Here's how the part is built. I have some questions about the finished solid (model axes, mm). Coordinates: 2 decimals unless noted, no trailing zeros. Loops run counter-clockwise (first coordinate to the right, second up) from the corner with the lowest first, then second, coordinate; pieces in that order, holes last.
from build123d import *

# Parameters (mm, degrees)
SKETCH1_W               = 70
SKETCH1_H               = 100
BOSS_EXTRUDE1_DEPTH     = 1
CUT_EXTRUDE1_DEPTH      = 62.040969848
CUT_EXTRUDE1_DEPTH_BACK = 62.040969848
SKETCH2_R               = 1.7


with BuildPart() as part:
    # Sketch1 → Boss-Extrude1 (new body)
    with BuildSketch(Plane.XY):
        Rectangle(SKETCH1_W, SKETCH1_H)
    extrude(amount=-BOSS_EXTRUDE1_DEPTH)

    # Sketch2 → Cut-Extrude1 (cut, two sides: drawn at the far end of the back side and taken through both)
    with BuildSketch(Plane.XY.offset(-CUT_EXTRUDE1_DEPTH_BACK)):
        with Locations((-30, -35)):
            Circle(SKETCH2_R)
        with Locations((-30, 35)):
            Circle(SKETCH2_R)
        with Locations((30, -35)):
            Circle(SKETCH2_R)
        with Locations((30, 35)):
            Circle(SKETCH2_R)
        with Locations((-15, -40)):
            Circle(SKETCH2_R)
        with Locations((-15, -10)):
            Circle(SKETCH2_R)
        with Locations((-15, 10)):
            Circle(SKETCH2_R)
        with Locations((-15, 40)):
            Circle(SKETCH2_R)
        with Locations((15, -40)):
            Circle(SKETCH2_R)
        with Locations((15, -10)):
            Circle(SKETCH2_R)
        with Locations((15, 10)):
            Circle(SKETCH2_R)
        with Locations((15, 40)):
            Circle(SKETCH2_R)
    extrude(amount=CUT_EXTRUDE1_DEPTH + CUT_EXTRUDE1_DEPTH_BACK, mode=Mode.SUBTRACT)


solid = part.part
Q1. Suppose I cut it at A-A on x = 30. Write out the boundary of the cut face in (y, z), and give its area (3 significant figures).
Q2. Suppose I cut it at B-B on z = -0.7. State how many separate pieces and enclosed holes the cut face has, and give its area (3 significant figures).
Q3. Will this pin go through, and if not, where does the flat tip stop? P1, Ø2.5, axis at x = -15, y = -40, coming from the -Z side.
Q4. Suppose I cut it at C-C on y = 35. Write out the boundary of the cut face in (x, z).
Q5. We'd pull the mould along Y, two halves only. Please class faces 1 (the flat face through (0, 1, -1)), 2 (the cylindrical face through (30.8, 33.5, -0.5)): pulls with the +Y half, pulls with the -Y half, needs draft (parallel to the pull), parting line crosses it, or undercut.
Q6. Suppose I cut it at D-D on x = 15. Write out the boundary of the cut face in (y, z), and give its area (3 significant figures).
Q7. Please list where these lines run through material, in increasing order: probe 1 along Y at (x, z) = (30, -0.4); probe 2 along X at (y, z) = (35, -0.55); probe 3 along Y at (x, z) = (-15, -0.25).
Check values:
1. outline: (-50, -1) - (-36.7, -1) - (-36.7, 0) - (-50, 0) - close; (-33.3, -1) - (33.3, -1) - (33.3, 0) - (-33.3, 0) - close; (36.7, -1) - (50, -1) - (50, 0) - (36.7, 0) - close
1. area: 93.2 mm2
2. separate pieces: 1
2. enclosed holes: 12
2. area: 6,890 mm2
3. P1: passes through
4. outline: (-35, -1) - (-31.7, -1) - (-31.7, 0) - (-35, 0) - close; (-28.3, -1) - (28.3, -1) - (28.3, 0) - (-28.3, 0) - close; (31.7, -1) - (35, -1) - (35, 0) - (31.7, 0) - close
5. face 1: needs draft
5. face 2: undercut
6. outline: (-50, -1) - (-41.7, -1) - (-41.7, 0) - (-50, 0) - close; (-38.3, -1) - (-11.7, -1) - (-11.7, 0) - (-38.3, 0) - close; (-8.3, -1) - (8.3, -1) - (8.3, 0) - (-8.3, 0) - close; (11.7, -1) - (38.3, -1) - (38.3, 0) - (11.7, 0) - close; (41.7, -1) - (50, -1) - (50, 0) - (41.7, 0) - close
6. area: 86.4 mm2
7. probe 1: y = -50 to -36.7, -33.3 to 33.3, 36.7 to 50
7. probe 2: x = -35 to -31.7, -28.3 to 28.3, 31.7 to 35
7. probe 3: y = -50 to -41.7, -38.3 to -11.7, -8.3 to 8.3, 11.7 to 38.3, 41.7 to 50
